from build123d import *

# Parameters (mm, degrees)
SKETCH1_R           = 4
BOSS_EXTRUDE1_DEPTH = 15
SKETCH2_W           = 5.6
SKETCH2_H           = 3.95
CUT_EXTRUDE1_DEPTH  = 8
CUT_EXTRUDE2_DEPTH  = 7


with BuildPart() as part:
    # Sketch1 → Boss-Extrude1 (new body)
    with BuildSketch(Plane.XY):
        Circle(SKETCH1_R)
    extrude(amount=BOSS_EXTRUDE1_DEPTH)

    # Sketch2 → Cut-Extrude1 (cut)
    with BuildSketch(Plane.XY.offset(15)):
        Rectangle(SKETCH2_W, SKETCH2_H)
    extrude(amount=-CUT_EXTRUDE1_DEPTH, mode=Mode.SUBTRACT)

    # Sketch3 → Cut-Extrude2 (cut)
    with BuildSketch(Plane(origin=(0, 0, 0), x_dir=(-1, 0, 0), z_dir=(0, 0, -1))):
        with BuildLine():
            Line((0.948044642, -2.451135369), (0.948044642, -1.45))
            ThreePointArc((0.948044642, -1.45), (1.145326424, -1.147281782), (1.448044642, -0.95))
            Line((1.448044642, -0.95), (2.446909273, -0.95))
            ThreePointArc((2.446909273, -0.95), (2.561359119, 0), (2.446909273, 0.95))
            Line((2.446909273, 0.95), (1.445773904, 0.95))
            ThreePointArc((1.445773904, 0.95), (1.137533058, 1.141759153), (0.945773904, 1.45))
            Line((0.945773904, 1.45), (0.945773904, 2.448864631))
            ThreePointArc((0.945773904, 2.448864631), (-0.004226096, 2.563314477), (-0.954226096, 2.448864631))
            Line((-0.954226096, 2.448864631), (-0.954226096, 1.447729262))
            ThreePointArc((-0.954226096, 1.447729262), (-1.145985249, 1.139488415), (-1.454226096, 0.947729262))
            Line((-1.454226096, 0.947729262), (-2.453090727, 0.947729262))
            ThreePointArc((-2.453090727, 0.947729262), (-2.567540573, -0.002270738), (-2.453090727, -0.952270738))
            Line((-2.453090727, -0.952270738), (-1.451955358, -0.952270738))
            ThreePointArc((-1.451955358, -0.952270738), (-1.143714511, -1.144029891), (-0.951955358, -1.452270738))
            Line((-0.951955358, -1.452270738), (-0.951955358, -2.451135369))
            ThreePointArc((-0.951955358, -2.451135369), (-0.001955358, -2.565585215), (0.948044642, -2.451135369))
        make_face()
    extrude(amount=-CUT_EXTRUDE2_DEPTH, mode=Mode.SUBTRACT)


solid = part.part
The listing builds one solid part. Answer for the finished solid, in the listing's coordinates (mm). A direction names the side the tool comes from. Coordinates: 2 decimals unless noted, no trailing zeros. Loops run counter-clockwise (first coordinate to the right, second up) from the corner with the lowest first, then second, coordinate; pieces in that order, holes last.
1) Find section C-C on z = 3.75. Write down the section's boundary in (x, y).
2) Flat-ended cylindrical pins translate along their axes: pin 1 Ø1 at (x, z) = (1, 12.5) entering from +Y; pin 2 Ø0.5 at (x, z) = (-2, 2.5) entering from +Y; pin 3 Ø0.8 at (y, z) = (-1.5, 2.5) entering from +X; pin 4 Ø0.6 at (x, y) = (-2, 0) entering from +Z. Find the tip coordinate at first contact, or state that the pin passes through.
3) A tool of negligible diameter and unlimited length cuts with its end or side. For faces 5 (the face through (-2.8, 0, 11)), 6 (the face through (2.568, 0.011, 3.451)), 7 (the face through (-0.009, 2.563, 3.451)), from which of +Z, -Z, +X, -X, +Y, -Y can it reach the whole face along a straight path? Write none if from no direction.
4) Find section D-D on z = 8.25. Write down the section's boundary in (x, y) (3 decimals).
5) Find section A-A on x = 0. Write down the section's boundary in (y, z) (3 decimals), then the cut area to 3 significant figures.
6) Determine the mould class of faces 1 (the face through (2, -2, 0)), 2 (the face through (2, 0.948, 3)), 3 (the face through (0.954, 2, 3)), 4 (the face through (-0.867, -3.905, 7.395)) for opening direction Y: pulls with the +Y half, pulls with the -Y half, needs draft (parallel to the pull), parting line crosses it, or undercut.
7) Find section B-B on y = 0. Write down the section's boundary in (x, z).
8) Find the intervals of material crossed by L1, parallel to X at y = -0.75, z = 10.5; L2, parallel to Y at x = 2.25, z = 3.25; L3, parallel to X at y = -2, z = 1.25, in increasing order.
Values:
1. outline: circle Ø8 at (0, 0); hole (-2.45, -0.95) - (-1.45, -0.95) arc R0.88 cw to (-0.95, -1.45) - (-0.95, -2.45) arc R4 ccw to (0.95, -2.45) - (0.95, -1.45) arc R0.8 cw to (1.45, -0.95) - (2.45, -0.95) arc R4 ccw to (2.45, 0.95) - (1.45, 0.95) arc R0.8 cw to (0.95, 1.45) - (0.95, 2.45) arc R4 ccw to (-0.95, 2.45) - (-0.95, 1.45) arc R0.8 cw to (-1.45, 0.95) - (-2.45, 0.95) arc R4 ccw to start
2. pin 1: stops at y = 3.97
2. pin 2: stops at y = 3.6
2. pin 3: stops at x = 3.85
2. pin 4: passes through
3. face 5: +Z
3. face 6: +Z, -Z
3. face 7: -Z
4. outline: circle Ø8 at (0, 0); hole (-2.8, -1.975) - (2.8, -1.975) - (2.8, 1.975) - (-2.8, 1.975) - close
5. outline: (-4, 0) - (-2.566, 0) - (-2.566, 7) - (-1.975, 7) - (-1.975, 15) - (-4, 15) - close; (1.975, 7) - (2.563, 7) - (2.563, 0) - (4, 0) - (4, 15) - (1.975, 15) - close
5. area: 52.5 mm2
6. face 1: needs draft
6. face 2: undercut
6. face 3: undercut
6. face 4: parting line crosses it
7. outline: (-4, 0) - (-2.56, 0) - (-2.56, 7) - (-2.8, 7) - (-2.8, 15) - (-4, 15) - close; (2.57, 0) - (4, 0) - (4, 15) - (2.8, 15) - (2.8, 7) - (2.57, 7) - close
8. L1: x = -3.93 to -2.8, 2.8 to 3.93
8. L2: y = -3.31 to -0.95, 0.95 to 3.31
8. L3: x = -3.46 to -0.95, 0.95 to 3.46
